Read the model definition and answer for the solid it produces. Units are mm, in the model's axes. A direction names the side the tool comes from. Give positions to 0.01 mm unless a question says otherwise; leave off trailing zeros. Write each loop counter-clockwise with the first axis right and the second up, starting at its lowest first coordinate (ties: lowest second). Pieces come first, ordered by that corner, then holes. Notation, with made-up numbers: M 32,86.5 L 85,86.5 A28 ccw 85,105.5 Z; hole C 51,27 d1. An arc over 180 degrees is marked long. Answer as CSV lines item,"result". Start each with the question number.
```python
from build123d import *

# Parameters (mm, degrees)
F1_DEPTH = 15
F2_W     = 15
F2_H     = 25
F3_DEPTH = 15


with BuildPart() as f1:
    # F0 (on Front) → F1 (new body, symmetric)
    with BuildSketch(Plane.XZ):
        Polygon((0, 35), (0, 0), (40, 0), (40, 10), (15, 10), (15, 35), align=None)
    extrude(amount=F1_DEPTH, both=True)

    # F2 (on Front) → F3 (join)
    with BuildSketch(Plane.XZ):
        with Locations((22.5, 22.5)):
            Rectangle(F2_W, F2_H)
    extrude(amount=-F3_DEPTH)


solid = f1.part
```
1. Find section C-C on x = 31.5. Determine the outline of the cut face in (y, z), then the cut area to 3 significant figures.
2. Given pin 1 (12 mm diameter, centred on y = -9.5, z = 20.5, fed in from +X); pin 2 (12 mm diameter, centred on y = 5.5, z = 23, fed in from +X); pin 3 (12 mm diameter, centred on x = 23, z = 18.5, fed in from -Y), each flat-ended and moving along its own axis, determine where each tip first touches the part or whether it passes through.
3. Find the intervals of material crossed by line 1 (Y direction, x = 17, z = 28.5); line 2 (Z direction, x = 28.5, y = -11.5), in increasing order. Write a range as [from, to].
4. Find section B-B on x = 23.5. Determine the outline of the cut face in (y, z), then the cut area to 3 significant figures.
5. Find section A-A on y = 9.75. Determine the outline of the cut face in (x, z).
6. For faces 1 (the face through (30, 7, 22)), 2 (the face through (22, 0, 23)), 3 (the face through (0, 0, 18)), determine the directions among +Z, -Z, +X, -X, +Y, -Y from which every point of the face is accessible in a straight line to the end or side of a thin tool.
Computed:
1,outline,"M -15,0 L 15,0 L 15,10 L -15,10 Z"
1,area,"300 mm^2"
2,pin 1,"stops at x = 15"
2,pin 2,"stops at x = 30"
2,pin 3,"stops at y = 0"
3,line 1,"y = [0, 15]"
3,line 2,"z = [0, 10]"
4,outline,"M -15,0 L 15,0 L 15,35 L 0,35 L 0,10 L -15,10 Z"
4,area,"675 mm^2"
5,outline,"M 0,0 L 40,0 L 40,10 L 30,10 L 30,35 L 0,35 Z"
6,face 1,"+Z, +X, +Y, -Y"
6,face 2,"+Z, +X, -Y"
6,face 3,"+Z, -Z, -X, +Y, -Y"
